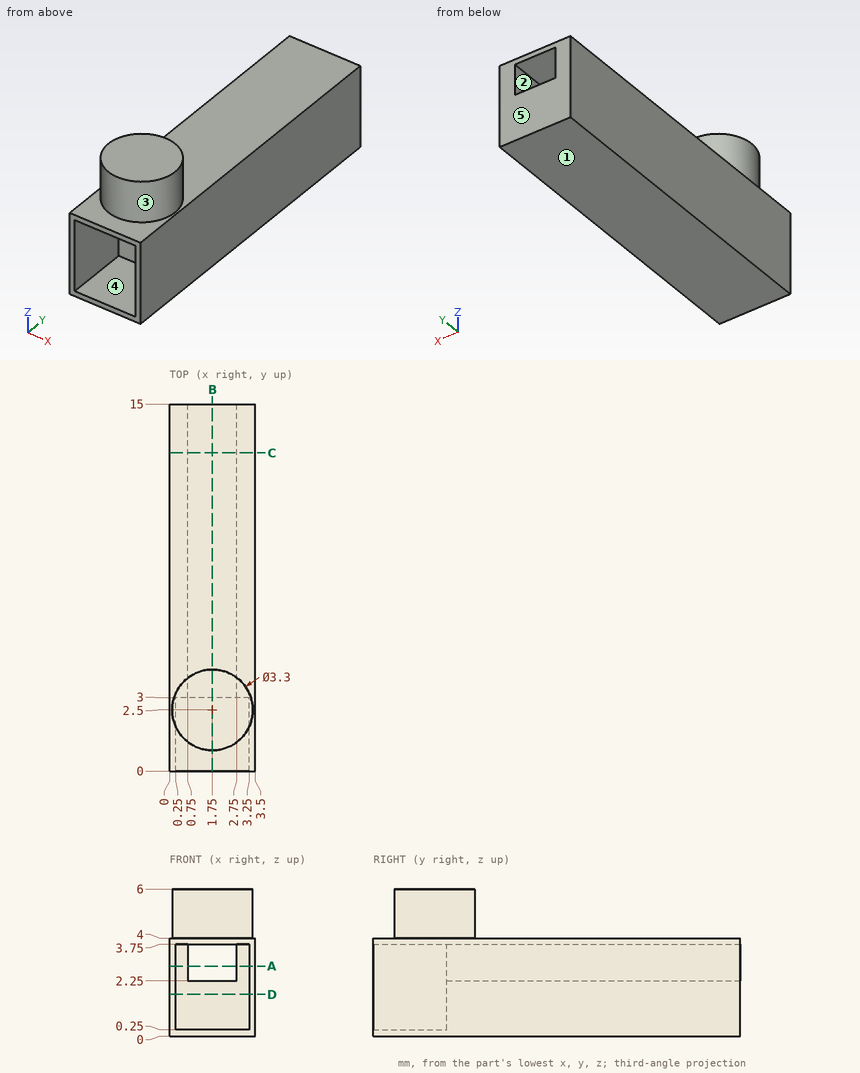
Input: dimensioned drawing with shaded views. Units: mm. Origin: part minimum x, y, z. A direction names the side the tool comes from. Give positions to 0.01 mm unless a question says otherwise; leave off trailing zeros. Write each loop counter-clockwise with the first axis right and the second up, starting at its lowest first coordinate (ties: lowest second). Pieces come first, ordered by that corner, then holes.
1. Section query A-A, the plane z = 2.85. Return loops of the section in (x, y), then the cut area to 3 significant figures.
2. Section query D-D, the plane z = 1.7. Return loops of the section in (x, y).
3. Pin query (flat end, axial travel): P1, Ø1, axis at y = 1.5, z = 4, coming from the -X side; P2, Ø1, axis at x = 1.5, y = 6, coming from the +Z side. Return the tip coordinate at first contact, or that it passes through.
4. Reachability of the marked faces 4 and 5 from +Z, -Z, +X, -X, +Y, -Y: full face, straight path, thin tool, end or side. Return the list, or none.
5. Section query C-C, the plane y = 13. Return loops of the section in (x, z).
6. Line query: probe 1 along Z at (x, y) = (1.4, 9.25); probe 2 along Z at (x, y) = (0.45, 2); probe 3 along Y at (x, z) = (1.15, 1.35). Output: solid intervals per line, ascending.
7. Draft query along X for the marked faces 1, 2 and 3. Return one class per face: released by +X, released by -X, zero draft, split by the parting line, or undercut.
8. Section query B-B, the plane x = 1.75. Return loops of the section in (y, z), then the cut area to 3 significant figures.
Computed:
1. outline: (0, 0) - (0.25, 0) - (0.25, 3) - (0.75, 3) - (0.75, 15) - (0, 15) - close; (2.75, 3) - (3.25, 3) - (3.25, 0) - (3.5, 0) - (3.5, 15) - (2.75, 15) - close
1. area: 19.5 mm2
2. outline: (0, 0) - (0.25, 0) - (0.25, 3) - (3.25, 3) - (3.25, 0) - (3.5, 0) - (3.5, 15) - (0, 15) - close
3. P1: stops at x = 0
3. P2: stops at z = 4
4. face 4: -Y
4. face 5: +Z, -Z, +X, -X, +Y
5. outline: (0, 0) - (3.5, 0) - (3.5, 4) - (0, 4) - close; hole (0.75, 2.25) - (2.75, 2.25) - (2.75, 3.75) - (0.75, 3.75) - close
6. probe 1: z = 0 to 2.25, 3.75 to 4
6. probe 2: z = 0 to 0.25, 3.75 to 6
6. probe 3: y = 3 to 15
7. face 1: zero draft
7. face 2: undercut
7. face 3: split by the parting line
8. outline: (0, 0) - (15, 0) - (15, 2.25) - (3, 2.25) - (3, 0.25) - (0, 0.25) - close; (0, 3.75) - (15, 3.75) - (15, 4) - (4.15, 4) - (4.15, 6) - (0.85, 6) - (0.85, 4) - (0, 4) - close
8. area: 38.1 mm2
